The drawing under review shows one solid part. Ordinate dimensions are in mm from its lowest x, y, z. A direction names the side the tool comes from. Round coordinates to 2 decimals unless told otherwise and drop trailing zeros. Order: outer loops, then holes, each group sorted by start corner. A loop starts at its lowest first (then second) coordinate and runs counter-clockwise, first axis right, second up. Notation, with made-up numbers: (-2, 88.25) -> (19, 88.25) arc R31 ccw to (19, 116.25) -> close; hole circle Ø2 at (-28.5, 58). An arc over 180 degrees is marked (long way). Use a Markdown table: item, result. Add a question column.
1) Draft analysis for pull direction Y (two halves, no side actions). For the marked faces 3, 4 and 5, state which applies: pulls with the +Y half, pulls with the -Y half, needs draft (parallel to the pull), parting line crosses it, or undercut.
2) Consider section B-B (z = 7.25). State the section outline as (x, y) points, plus the area to 3 significant figures.
3) Wall thickness on line 1 along Y through (x, z) = (4, 6.25); line 2 along Y through (x, z) = (21, 5); line 3 along X through (y, z) = (4.25, 1.5): over which ranges is each line inside the solid? List them lowest first. Write a range as [from, to].
4) Consider section C-C (y = 4). State the section outline as (x, z) points.
5) Consider section D-D (z = 1). State the section outline as (x, y) points.
6) Clearance check with a flat-ended pin moving along its axis: P1, Ø1, axis at x = 27, y = 2, coming from the +Z side. State where the tip first meets the part, or that it passes through.
7) Machinability: for the marked faces 1 and 2, which of the approach directions +Z, -Z, +X, -X, +Y, -Y give a long, thin tool a straight path to every point of the face, cutting with its end or side? Answer none if there is none.
8) Consider section A-A (x = 36). State the section outline as (y, z) points, plus the area to 3 significant figures.
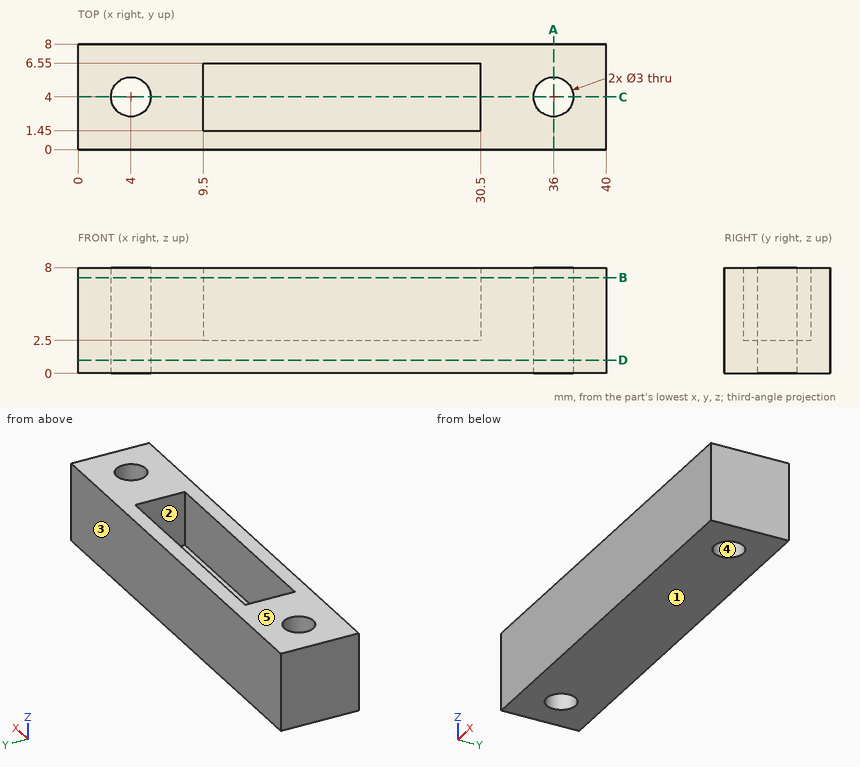
Results list:
| question | item | result |
|---|---|---|
| 1 | face 3 | pulls with the +Y half |
| 1 | face 4 | undercut |
| 1 | face 5 | needs draft |
| 2 | outline | (0, 0) -> (40, 0) -> (40, 8) -> (0, 8) -> close; hole circle Ø3 at (4, 4); hole (9.5, 1.45) -> (30.5, 1.45) -> (30.5, 6.55) -> (9.5, 6.55) -> close; hole circle Ø3 at (36, 4) |
| 2 | area | 199 mm2 |
| 3 | line 1 | [0, 2.5], [5.5, 8] |
| 3 | line 2 | [0, 1.45], [6.55, 8] |
| 3 | line 3 | [0, 2.52], [5.48, 34.52], [37.48, 40] |
| 4 | outline | (0, 0) -> (2.5, 0) -> (2.5, 8) -> (0, 8) -> close; (5.5, 0) -> (34.5, 0) -> (34.5, 8) -> (30.5, 8) -> (30.5, 2.5) -> (9.5, 2.5) -> (9.5, 8) -> (5.5, 8) -> close; (37.5, 0) -> (40, 0) -> (40, 8) -> (37.5, 8) -> close |
| 5 | outline | (0, 0) -> (40, 0) -> (40, 8) -> (0, 8) -> close; hole circle Ø3 at (4, 4); hole circle Ø3 at (36, 4) |
| 6 | P1 | z = 2.5 |
| 7 | face 1 | -Z, +X, -X, +Y, -Y |
| 7 | face 2 | +Z |
| 8 | outline | (0, 0) -> (2.5, 0) -> (2.5, 8) -> (0, 8) -> close; (5.5, 0) -> (8, 0) -> (8, 8) -> (5.5, 8) -> close |
| 8 | area | 40.0 mm2 |
